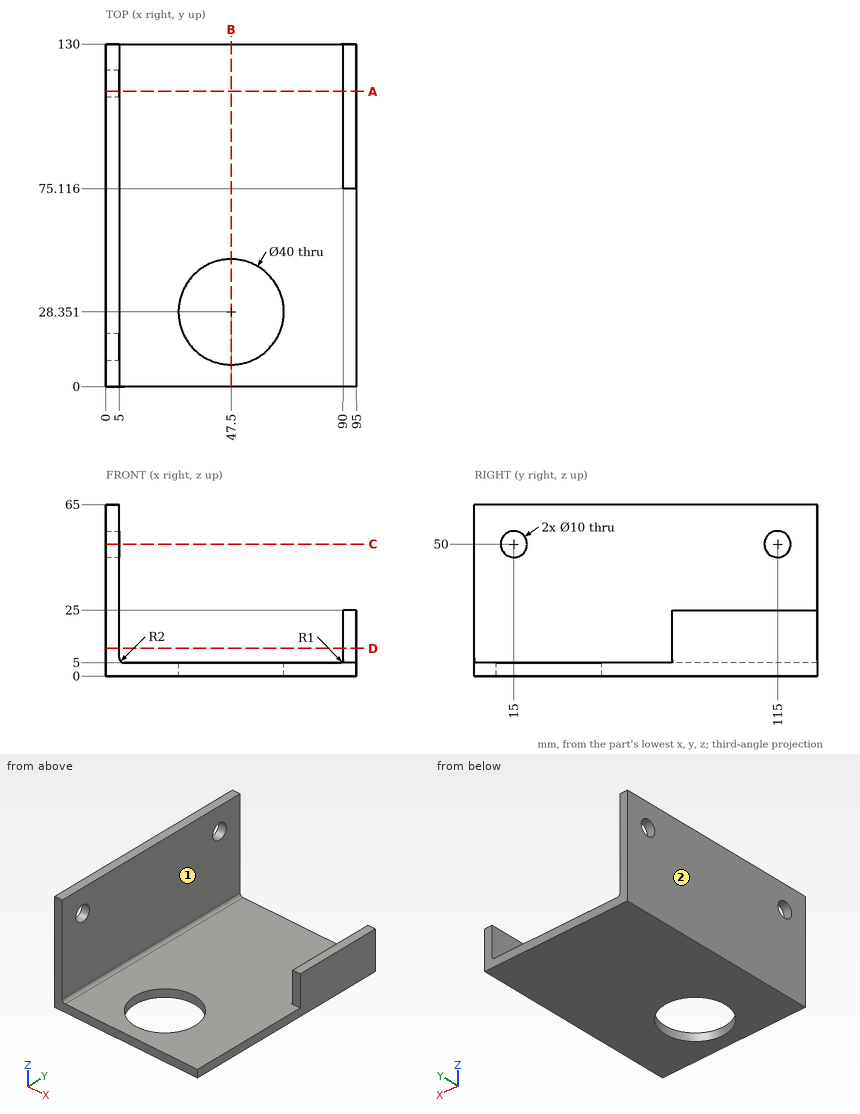
Job drawing, mm, ordinate dimensions from the low corner. One solid piece. A direction names the side the tool comes from. Round coordinates to 2 decimals unless told otherwise and drop trailing zeros. Loops run counter-clockwise (first coordinate to the right, second up) from the corner with the lowest first, then second, coordinate; pieces in that order, holes last. Notation, with made-up numbers: (3.25, -30.5) -> (54.25, -30.5) arc R25 cw to (54.25, -9.5) -> close; hole circle Ø2 at (-5, 77.25). An arc over 180 degrees is marked (long way). One line per item, written item: value. Start each with the question number.
Q1. Cut at A-A on y = 112. List the corners of the cut face in (x, z).
Q2. Drop flat-ended pins along their axis: pin 1 Ø8 at (y, z) = (115, 50) entering from +X; pin 2 Ø6.5 at (x, z) = (91, 15.5) entering from -Y; pin 3 Ø4 at (x, y) = (92.5, 113.5) entering from +Z; pin 4 Ø12 at (x, y) = (32, 56) entering from +Z. Give the stop position or say it passes through.
Q3. 3-axis set-ups, long thin cutter, end or side, ignore diameter. For the marked faces 1 and 2: which of +Z, -Z, +X, -X, +Y, -Y reach the whole face in a straight line?
Q4. Cut at B-B on x = 47.5. List the corners of the cut face in (y, z).
Q5. Cut at D-D on z = 10.5. List the corners of the cut face in (x, y).
Q6. Cut at C-C on z = 50. List the corners of the cut face in (x, y), plus the area to 3 significant figures.
Q7. Probe line 1 along Z through (x, y) = (3.25, 115); line 2 along Z through (x, y) = (89, 100). List the from-to ranges inside material, lowest first.
Computed:
1. outline: (0, 0) -> (95, 0) -> (95, 25) -> (90, 25) -> (90, 6) arc R1 cw to (89, 5) -> (7, 5) arc R2 cw to (5, 7) -> (5, 46) -> (0, 46) -> close; (0, 54) -> (5, 54) -> (5, 65) -> (0, 65) -> close
2. pin 1: through
2. pin 2: y = 75.12
2. pin 3: z = 25
2. pin 4: z = 5
3. face 1: +Z, +Y, -Y
3. face 2: +Z, -Z, -X, +Y, -Y
4. outline: (0, 0) -> (8.35, 0) -> (8.35, 5) -> (0, 5) -> close; (48.35, 0) -> (130, 0) -> (130, 5) -> (48.35, 5) -> close
5. outline: (0, 0) -> (5, 0) -> (5, 130) -> (0, 130) -> close; (90, 75.12) -> (95, 75.12) -> (95, 130) -> (90, 130) -> close
6. outline: (0, 0) -> (5, 0) -> (5, 10) -> (0, 10) -> close; (0, 20) -> (5, 20) -> (5, 110) -> (0, 110) -> close; (0, 120) -> (5, 120) -> (5, 130) -> (0, 130) -> close
6. area: 550 mm²
7. line 1: 0 to 45, 55 to 65
7. line 2: 0 to 5
